Source: CAD feature listing. Evaluate the final solid. Frame: model axes, mm. A direction names the side the tool comes from. Give positions to 0.01 mm unless a question says otherwise; leave off trailing zeros. Order: outer loops, then holes, each group sorted by start corner. A loop starts at its lowest first (then second) coordinate and runs counter-clockwise, first axis right, second up. Notation, with made-up numbers: M -28.5,58 L -17.5,58 A26 cw -17.5,86 Z; hole C 48,-14 d7. An arc over 180 degrees is marked long. Return JSON: item names as keys, results as strings.
from build123d import *

# Parameters (mm, degrees)
SALIENTE_EXTRUIR1_DEPTH = 30


with BuildPart() as part:
    # Croquis1 → Saliente-Extruir1 (new body)
    with BuildSketch(Plane(origin=(0, 0, 0), x_dir=(1, 0, 0), z_dir=(0, 1, 0))):
        Polygon((300, -124.264068712), (300, 124.264068712), (124.264068712, 300), (-124.264068712, 300), (-300, 124.264068712), (-300, -124.264068712), (-124.264068712, -300), (124.264068712, -300), align=None)
        Polygon((270, -111.837661841), (270, 111.837661841), (111.837661841, 270), (-111.837661841, 270), (-270, 111.837661841), (-270, -111.837661841), (-111.837661841, -270), (111.837661841, -270), align=None, mode=Mode.SUBTRACT)
    extrude(amount=SALIENTE_EXTRUIR1_DEPTH)


solid = part.part
1. Draft query along X for faces 1 (the face through (-2, 15, 300)), 2 (the face through (-2, 15, 270)), 3 (the face through (-189.81, 14.79, -192.03)), 4 (the face through (-210.902, 14.79, -213.362)). Return one class per face: pulls with the +X half, pulls with the -X half, needs draft (parallel to the pull), parting line crosses it, or undercut.
Evaluation:
{"face 1": "needs draft", "face 2": "undercut", "face 3": "undercut", "face 4": "pulls with the -X half"}
2. Section query B-B (z = 172). Return loops of the section in (x, y).
Evaluation:
{"outline": "M -252.26,0 L -209.84,0 L -209.84,30 L -252.26,30 Z; M 209.84,0 L 252.26,0 L 252.26,30 L 209.84,30 Z"}
3. Ray query, probe 1 along Z at (x, y) = (58, 2.75); probe 2 along X at (y, z) = (12.5, 169). Return the intervals inside material, ascending.
Evaluation:
{"probe 1": "z = -300 to -270, 270 to 300", "probe 2": "x = -255.26 to -212.84, 212.84 to 255.26"}
4. Section query A-A (x = -88.5). Return loops of the section in (y, z), then the cut area to 3 significant figures.
Evaluation:
{"outline": "M 0,-300 L 30,-300 L 30,-270 L 0,-270 Z; M 0,270 L 30,270 L 30,300 L 0,300 Z", "area": "1,800 mm^2"}
5. First-contact query: pin 1 (3 mm diameter, centred on y = 14, z = 219.5, fed in from -X); pin 2 (3 mm diameter, centred on y = 23.5, z = 193.5, fed in from -X); pin 3 (1.5 mm diameter, centred on x = -236, y = 8.5, fed in from -Z). Flat tips, straight axial feed; report the tip coordinate or a pass-through.
Evaluation:
{"pin 1": "stops at x = -206.26", "pin 2": "stops at x = -232.26", "pin 3": "stops at z = -189.01"}
6. Set-up query: faces 5 (the face through (192.03, 14.79, -189.81)), 6 (the face through (210.902, 14.79, 213.362)). Return all of +Z, -Z, +X, -X, +Y, -Y with unobstructed straight access to the full face (end or side cutting, diameter ignored); none if empty.
Evaluation:
{"face 5": "+Y, -Y", "face 6": "+Z, +X, +Y, -Y"}
7. Section query C-C (y = 18.5). Return loops of the section in (x, z).
Evaluation:
{"outline": "M -300,-124.26 L -124.26,-300 L 124.26,-300 L 300,-124.26 L 300,124.26 L 124.26,300 L -124.26,300 L -300,124.26 Z; hole M -270,-111.84 L -111.84,-270 L 111.84,-270 L 270,-111.84 L 270,111.84 L 111.84,270 L -111.84,270 L -270,111.84 Z"}
